Build history of the part. All positions in model axes, mm. A direction names the side the tool comes from. Round coordinates to 2 decimals unless told otherwise and drop trailing zeros. Write each loop counter-clockwise with the first axis right and the second up, starting at its lowest first coordinate (ties: lowest second). Pieces come first, ordered by that corner, then holes. Notation, with made-up numbers: M 8,72.25 L 26,72.25 A37 cw 26,111.25 Z; hole C 25,89.25 d11. An arc over 180 degrees is marked long. Write item = value, one per line. Start each with the question number.
Q1. Band-saw the part on D-D on z = 16.5. Write the cut outline in (x, y).
Q2. Pull direction X, two halves, no side cores. Call faces 1 (the cylindrical face through (-28.97, 1.47, 12.16)), 2 (the cylindrical face through (14.536, 4.578, 8.766)), 3 (the cylindrical face through (13.69, -4.31, 8.64)): released by +X, released by -X, zero draft, split by the parting line, or undercut.
Q3. Drop flat-ended pins along their axis: P1, Ø1.5, axis at y = 10.5, z = 3, coming from the +X side; P2, Ø10, axis at x = -21.5, z = 8.5, coming from the +Y side (3 decimals); P3, Ø4, axis at y = -10, z = 2, coming from the +X side. Give the stop position or say it passes through.
Q4. Probe L1, parallel to Z at x = -30.5, y = 0; L2, parallel to Y at x = 0, z = 10.75; L3, parallel to Y at x = 0, z = 17.7. List the from-to ranges inside material, lowest first.
Q5. Band-saw the part on A-A on y = 0. Write the cut outline in (x, z).
Q6. Tool access for faces 4 (the cylindrical face through (-28.132, -1.498, 11.696)), 5 (the flat face through (5.6, -13.5, 0)), 6 (the cylindrical face through (-13.39, -0.688, 6.247)): list every direction of +Z, -Z, +X, -X, +Y, -Y with a clear straight run to the whole face (end or side of a thin tool).
Q7. Band-saw the part on B-B on x = 0. Write the cut outline in (y, z).
Q8. Band-saw the part on C-C on z = 7.25. Write the cut outline in (x, y).
```python
from build123d import *

# Parameters (mm, degrees)
F0_R       = 15.24
F1_DEPTH   = 17.78
F2_R       = 14.351
F3_DEPTH   = 17.526
F5_R       = 3.175
F6_DEPTH   = 25.1968
F6_FACE_R  = 3.175
F7_DEPTH   = 5.842
F8_R       = 2.786893
F9_DEPTH   = 33.5026
F12_R      = 13.97
F13_DEPTH  = 0.4572
F13_FACE_R = 13.97
F14_DEPTH  = 0.6096


with BuildPart() as f1:
    # F0 (on Top) → F1 (new body)
    with BuildSketch(Plane.XY):
        Circle(F0_R)
    extrude(amount=F1_DEPTH)

    # F2 (on face) → F3 (cut)
    with BuildSketch(Plane(origin=(0, 0, 0), x_dir=(1, 0, 0), z_dir=(0, 0, -1))):
        Circle(F2_R)
    extrude(amount=-F3_DEPTH, mode=Mode.SUBTRACT)

    # F5 (on offset) → F6 (join)
    with BuildSketch(Plane.YZ.offset(-37.592)):
        with Locations((0, 9.3463)):
            Circle(F5_R)
    extrude(amount=F6_DEPTH)

    # F6_face (on face) → F7 (join)
    with BuildSketch(Plane(origin=(-37.592, 0, 9.3463), x_dir=(0, 1, 0), z_dir=(-1, 0, 0))):
        Circle(F6_FACE_R)
    extrude(amount=F7_DEPTH)

    # F8 (on face) → F9 (cut)
    with BuildSketch(Plane(origin=(-43.434, 0, 0), x_dir=(0, -1, 0), z_dir=(-1, 0, 0))):
        with Locations((0, 9.3463)):
            Circle(F8_R)
    extrude(amount=-F9_DEPTH, mode=Mode.SUBTRACT)

    # F12 (on face) → F13 (join)
    with BuildSketch(Plane.XY.offset(17.78)):
        Circle(F12_R)
    extrude(amount=F13_DEPTH)

    # F13_face (on face) → F14 (cut)
    with BuildSketch(Plane.XY.offset(18.2372)):
        Circle(F13_FACE_R)
    extrude(amount=-F14_DEPTH, mode=Mode.SUBTRACT)


solid = f1.part
```
Conclusion:
q1.outline = C 0,0 d30.48; hole C 0,0 d28.7
q2.face_1 = zero draft
q2.face_2 = split by the parting line
q2.face_3 = undercut
q3.P1 = 11.71
q3.P2 = 3.175
q3.P3 = 12.97
q4.L1 = 6.17 to 6.56, 12.13 to 12.52
q4.L2 = -15.24 to -14.35, 14.35 to 15.24
q4.L3 = -15.24 to -13.97, 13.97 to 15.24
q5.outline = M -43.43,6.17 L -15.24,6.17 L -15.24,0 L -14.35,0 L -14.35,6.17 L -12.4,6.17 L -12.4,6.56 L -43.43,6.56 Z; M -43.43,12.13 L -12.4,12.13 L -12.4,12.52 L -14.35,12.52 L -14.35,17.53 L 14.35,17.53 L 14.35,0 L 15.24,0 L 15.24,17.78 L 13.97,17.78 L 13.97,17.63 L -13.97,17.63 L -13.97,17.78 L -15.24,17.78 L -15.24,12.52 L -43.43,12.52 Z
q6.face_4 = -X
q6.face_5 = -Z, +X, -X, +Y, -Y
q6.face_6 = none
q7.outline = M -15.24,0 L -14.35,0 L -14.35,17.53 L 14.35,17.53 L 14.35,0 L 15.24,0 L 15.24,17.78 L 13.97,17.78 L 13.97,17.63 L -13.97,17.63 L -13.97,17.78 L -15.24,17.78 Z
q8.outline = M -43.43,-2.38 L -15.05,-2.38 A15.24 ccw long -15.05,2.38 L -43.43,2.38 L -43.43,1.84 L -12.4,1.84 L -12.4,2.38 L -14.15,2.38 A14.35 cw long -14.15,-2.38 L -12.4,-2.38 L -12.4,-1.84 L -43.43,-1.84 Z
